Autodesk Inventor part; units mm, degrees
ref_plane "YZ Plane" through (0, 0, 0) normal (1, 0, 0) x (0, 1, 0)
ref_plane "XZ Plane" through (0, 0, 0) normal (0, 1, 0) x (-1, 0, 0)
ref_plane "XY Plane" through (0, 0, 0) normal (0, 0, 1) x (1, 0, 0)
sketch "Sketch1" plane through (0, 0, 0) normal (0, 1, 0) x (-1, 0, 0)
  circle A0 centre (0, 0) radius 16
  dimension "d0" = 32
extrude "Extrusion1" add sketch "Sketch1" along normal blind 5
sketch "Sketch2" plane through (0, 5, 0) normal (0, 1, 0) x (1, 0, 0)
  circle A0 centre (0, 0) radius 7.5
  dimension "d3" = 15
extrude "Extrusion2" add sketch "Sketch2" along normal blind 40
sketch "Sketch3" plane through (0, 0, 0) normal (0, -1, 0) x (1, 0, 0)
  circle A0 centre (0, 0) radius 12 construction
  point P0 (0, 12)
  point P1 (12, 0)
  point P2 (0, -12)
  point P3 (-12, 0)
  dimension "d6" = 24
hole "Hole1" at (0, 0, 12) at (12, 0, 0) at (0, 0, -12) at (-12, 0, 0) direction (0, 1, 0) diameter 3.5 end through all counterbore diameter 6 counterbore depth 3.1
sketch "Sketch4" plane through (0, 0, 0) normal (0, -1, 0) x (1, 0, 0)
  point P0 (0, 0)
  point P1 (0, 0)
hole "Hole2" at (0, 0, 0) direction (0, 1, 0) diameter 8 end through all
sketch "Sketch5" plane through (0, 0, 0) normal (0, -1, 0) x (1, 0, 0)
  circle A0 centre (0, 0) radius 5
  circle A1 centre (0, 0) radius 6
  dimension "d21" = 10
  dimension "d22" = 12
extrude "Extrusion3" cut sketch "Sketch5" against normal blind 0.2
chamfer "Chamfer1" distance 0.5 angle 45 1 edges at (-7.5, 45, 0)
properties part number "Łożysko liniowe z kołnierzem okrągłym LMF08UU-L" material "Stainless Steel"
Work out the finished part from the listing and answer in its coordinate system (mm). A direction names the side the tool comes from. Give positions to 0.01 mm unless a question says otherwise; leave off trailing zeros. Write each loop counter-clockwise with the first axis right and the second up, starting at its lowest first coordinate (ties: lowest second). Pieces come first, ordered by that corner, then holes. Notation, with made-up numbers: (49.25, -34) - (53.25, -34) arc R18 ccw to (53.25, -12) - close; hole circle Ø9 at (89.5, 2.5). An arc over 180 degrees is marked (long way). One line per item, written item: value. Start each with the question number.
1. Find section C-C (y = 27.5). Write down the section's boundary in (x, z), then the cut area to 3 significant figures.
2. For a pull along Z with two mould halves and no side action, classify faces 4 (the flat face through (3, 45, 3)), 5 (the cylindrical face through (1.8, 1.6, -9.6)), 6 (the cylindrical face through (3.47, 2.46, 15.62)) as +Z half, -Z half, draft (parallel to the pull), parting line (faces both ways), or undercut.
3. Given pin 1 (4.5 mm diameter, centred on x = 0, z = -12, fed in from +Y); pin 2 (2 mm diameter, centred on x = -12, z = 0, fed in from -Y); pin 3 (3 mm diameter, centred on x = -0.5, z = 13, fed in from -Y); pin 4 (9.5 mm diameter, centred on x = 0, z = -12, fed in from +Y), each flat-ended and moving along its own axis, determine where each tip first touches the part or whether it passes through.
4. Find section D-D (z = 0). State how many separate pieces and enclosed holes the cut face has, then the cut area to 3 significant figures.
5. For faces 1 (the cylindrical face through (-7.493, 24.474, 0.33)), 2 (the cylindrical face through (-0.526, 4.063, 10.331)), 3 (the flat face through (0, 3.1, 10)), determine the directions among +Z, -Z, +X, -X, +Y, -Y from which every point of the face is accessible in a straight line to the end or side of a thin tool.
6. Find section A-A (z = -12). Write down the section's boundary in (x, y).
7. Consider probe 1 along X at (y, z) = (11, 0); probe 2 along Y at (x, z) = (7, -11); probe 3 along Y at (x, z) = (1.5, 5). Determine where each line is inside the solid, lowest interval first.
8. Find section B-B (x = -12). Write down the section's boundary in (y, z).
Geometry results:
1. outline: circle Ø15 at (0, 0); hole circle Ø8 at (0, 0)
1. area: 126 mm2
2. face 4: draft
2. face 5: undercut
2. face 6: parting line
3. pin 1: y = 5
3. pin 2: through
3. pin 3: y = 3.1
3. pin 4: y = 44.75
4. separate pieces: 4
4. enclosed holes: 0
4. area: 349 mm2
5. face 1: +Y
5. face 2: +Y, -Y
5. face 3: -Y
6. outline: (-10.58, 0) - (-3, 0) - (-3, 3.1) - (-1.75, 3.1) - (-1.75, 5) - (-10.58, 5) - close; (1.75, 3.1) - (3, 3.1) - (3, 0) - (10.58, 0) - (10.58, 5) - (1.75, 5) - close
7. probe 1: -7.5 to -4, 4 to 7.5
7. probe 2: 0 to 5
7. probe 3: 0.2 to 45
8. outline: (0, -10.58) - (5, -10.58) - (5, -1.75) - (3.1, -1.75) - (3.1, -3) - (0, -3) - close; (0, 3) - (3.1, 3) - (3.1, 1.75) - (5, 1.75) - (5, 10.58) - (0, 10.58) - close
